Check sheet for the drawn part. Datum: minimum x, y, z corner. Units: mm. Round coordinates to 2 decimals unless told otherwise and drop trailing zeros. Write each loop counter-clockwise with the first axis right and the second up, starting at its lowest first coordinate (ties: lowest second). Pieces come first, ordered by that corner, then holes. Notation, with made-up numbers: M -33,-7 L -28,-7 A21 ccw -28,14 Z; hole C 28,-13.5 d10. An arc over 180 degrees is marked long. Use a Markdown table: item, result.
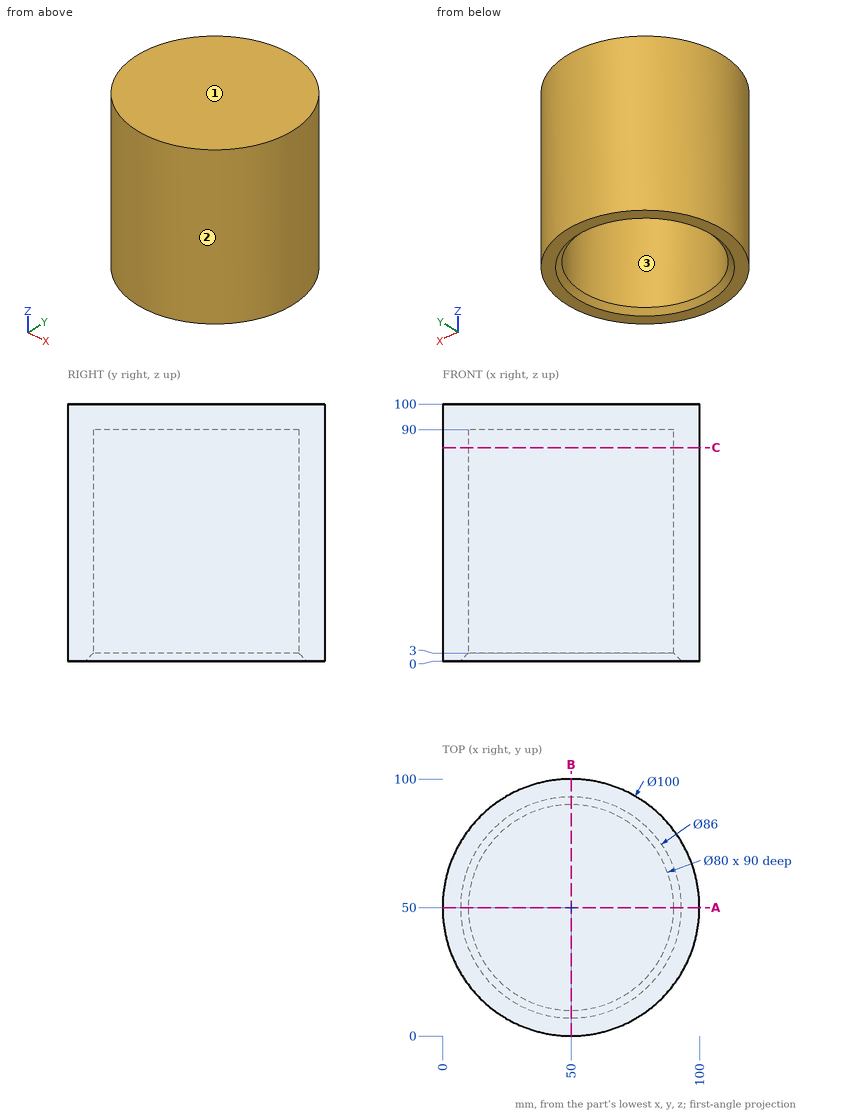
Item 1: Cross-section at A-A, the plane y = 50. Record the cut outline in (x, z), and give its area (3 significant figures).
Outcome:
| item | result |
|---|---|
| outline | M 0,0 L 7,0 L 10,3 L 10,90 L 90,90 L 90,3 L 93,0 L 100,0 L 100,100 L 0,100 Z |
| area | 2,790 mm2 |
Item 2: Mould release check, pull along X, two halves, no side actions. Record for the marked faces 1, 2 and 3: +X half, -X half, draft (parallel to the pull), parting line (faces both ways), or undercut.
Outcome:
| item | result |
|---|---|
| face 1 | draft |
| face 2 | parting line |
| face 3 | undercut |
Item 3: Cross-section at C-C, the plane z = 83. Record the cut outline in (x, y).
Outcome:
| item | result |
|---|---|
| outline | C 50,50 d100; hole C 50,50 d80 |
Item 4: Go/stop test with flat-tipped pins: pin 1 (4 mm diameter, centred on x = 41.5, y = 55, fed in from -Z); pin 2 (1 mm diameter, centred on y = 31.5, z = 72, fed in from +X); pin 3 (12 mm diameter, centred on x = 68.5, z = 82.5, fed in from -Y). Record where each tip stops, or that it passes through.
Outcome:
| item | result |
|---|---|
| pin 1 | stops at z = 90 |
| pin 2 | stops at x = 96.65 |
| pin 3 | stops at y = 1.59 |
Item 5: Material ranges on line 1 along Y through (x, z) = (50, 59); line 2 along Y through (x, z) = (65, 35.5); line 3 along X through (y, z) = (36, 31), recorded low to high. Write a range as from..to.
Outcome:
| item | result |
|---|---|
| line 1 | y = 0..10, 90..100 |
| line 2 | y = 2.3..12.92, 87.08..97.7 |
| line 3 | x = 2..12.53, 87.47..98 |
